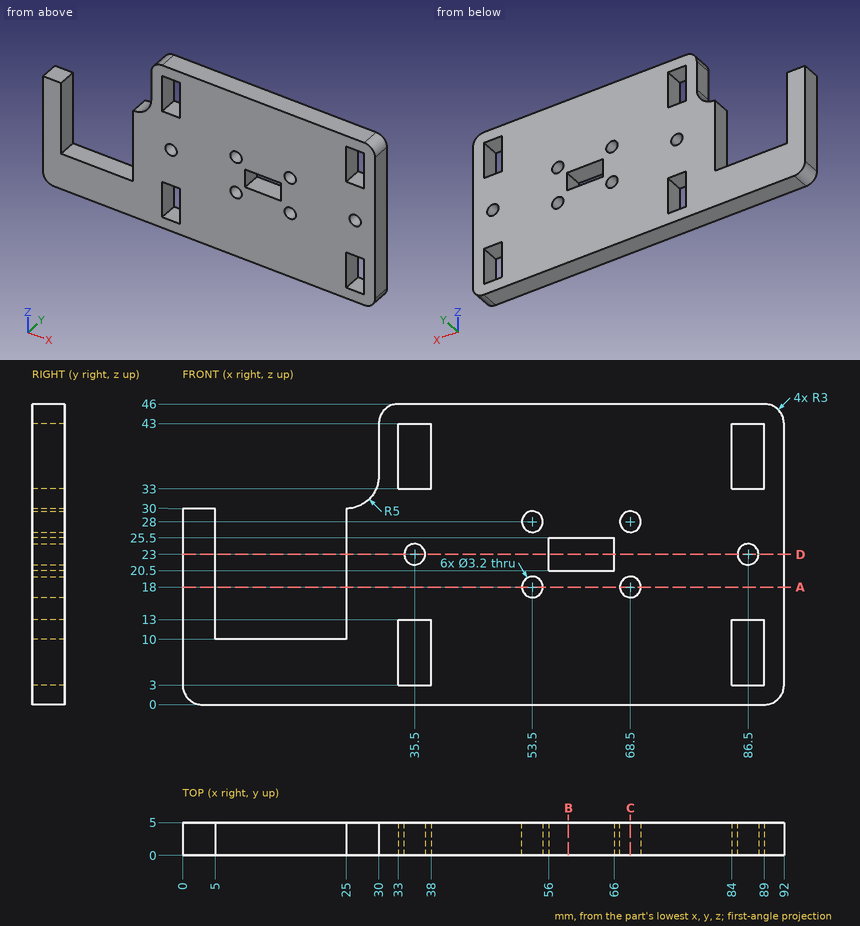
The drawing under review shows one solid part. Ordinate dimensions are in mm from its lowest x, y, z. Round coordinates to 2 decimals unless told otherwise and drop trailing zeros. Write each loop counter-clockwise with the first axis right and the second up, starting at its lowest first coordinate (ties: lowest second). Pieces come first, ordered by that corner, then holes. Notation, with made-up numbers: (8.5, 51) -> (48.5, 51) arc R32 cw to (48.5, 84) -> close; hole circle Ø7 at (-12.75, 63.5). An arc over 180 degrees is marked (long way). One line per question, with ' | ' between items. Start each with the question number.
(1) Add section B-B, the plane x = 59. Write out the cut boundary in (y, z), plus the area to 3 significant figures.
(2) Add section C-C, the plane x = 68.5. Write out the cut boundary in (y, z).
(3) Add section A-A, the plane z = 18. Write out the cut boundary in (x, y).
(4) For line 1 along X through (y, z) = (3.6, 11); line 2 along X through (y, z) = (3.8, 3.5); line 3 along X through (y, z) = (3.75, 25), list the stretches that pass through material, from the lowest coordinate up. Write a range as from..to.
(5) Insertion check: P1, Ø1.5, axis at x = 2.5, y = 2.5, coming from the +Z side; P2, Ø2.5, axis at x = 35.5, z = 23, coming from the +Y side; P3, Ø2.5, axis at y = 3, z = 41, coming from the -X side. Each pin has a flat end and moves straight along its axis. Give the tip position at first contact, or say it passes through.
(6) Add section D-D, the plane z = 23. Write out the cut boundary in (x, y), plus the area to 3 significant figures.
Answer list:
1) outline: (0, 0) -> (5, 0) -> (5, 20.5) -> (0, 20.5) -> close; (0, 25.5) -> (5, 25.5) -> (5, 46) -> (0, 46) -> close | area: 205 mm²
2) outline: (0, 0) -> (5, 0) -> (5, 16.4) -> (0, 16.4) -> close; (0, 19.6) -> (5, 19.6) -> (5, 26.4) -> (0, 26.4) -> close; (0, 29.6) -> (5, 29.6) -> (5, 46) -> (0, 46) -> close
3) outline: (0, 0) -> (5, 0) -> (5, 5) -> (0, 5) -> close; (25, 0) -> (51.9, 0) -> (51.9, 5) -> (25, 5) -> close; (55.1, 0) -> (66.9, 0) -> (66.9, 5) -> (55.1, 5) -> close; (70.1, 0) -> (92, 0) -> (92, 5) -> (70.1, 5) -> close
4) line 1: 0..5, 25..33, 38..84, 89..92 | line 2: 0..33, 38..84, 89..92 | line 3: 0..5, 25..56, 66..92
5) P1: z = 30 | P2: through | P3: x = 30
6) outline: (0, 0) -> (5, 0) -> (5, 5) -> (0, 5) -> close; (25, 0) -> (33.9, 0) -> (33.9, 5) -> (25, 5) -> close; (37.1, 0) -> (56, 0) -> (56, 5) -> (37.1, 5) -> close; (66, 0) -> (84.9, 0) -> (84.9, 5) -> (66, 5) -> close; (88.1, 0) -> (92, 0) -> (92, 5) -> (88.1, 5) -> close | area: 278 mm²
